from build123d import *

# Parameters (mm, degrees)
SKETCH_R           = 7
PAD_DEPTH          = 61
SKETCH001_R        = 5.425
POCKET_DEPTH       = 61.001
POCKET001_DEPTH    = 5
SKETCH004_W        = 4
SKETCH004_H        = 10
POCKET002_DEPTH    = 5
POLARPATTERN_COUNT = 4


with BuildPart() as part:
    # Sketch → Pad (new body)
    with BuildSketch(Plane.XY):
        Circle(SKETCH_R)
    extrude(amount=PAD_DEPTH)

    # Sketch001 (on Face3 of Pad) → Pocket (cut, through all)
    with BuildSketch(Plane.XY.offset(61)):
        Circle(SKETCH001_R)
    extrude(amount=-POCKET_DEPTH, mode=Mode.SUBTRACT)

    # Sketch002 (on DatumPlane) → Groove (revolve, cut)
    with BuildSketch(Plane(origin=(0, 0, 30.5), x_dir=(0, 0, -1), z_dir=(1, 0, 0))):
        Polygon((-8.25, 9.031089), (-11.75, 9.031089), (-10, 6), align=None)
    revolve(axis=Axis((0, 0, 0), (0, 0, 1)), mode=Mode.SUBTRACT)

    # Sketch003 (on DatumPlane) → Pocket001 (cut)
    with BuildSketch(Plane.YZ.offset(7)):
        Polygon((0, 4.732051), (-1.5, 2.133975), (1.5, 2.133975), align=None)
    extrude(amount=-POCKET001_DEPTH, mode=Mode.SUBTRACT)

    # Sketch004 (on DatumPlane) → Pocket002 (cut)
    with BuildSketch(Plane.YZ.offset(7)):
        with Locations((0, 40.5)):
            Rectangle(SKETCH004_W, SKETCH004_H)
    pocket002 = extrude(amount=-POCKET002_DEPTH, mode=Mode.SUBTRACT)

    # PolarPattern: Pocket002 ×4 about axis
    polarpattern_axis = Axis((0, 0, 0), (0, 0, 1))
    for i in range(1, POLARPATTERN_COUNT):
        add(pocket002.rotate(polarpattern_axis, i * 360 / POLARPATTERN_COUNT), mode=Mode.SUBTRACT)


solid = part.part
Model file for the job. Use its own axes, mm. A direction names the side the tool comes from. Give positions to 0.01 mm unless a question says otherwise; leave off trailing zeros. Write each loop counter-clockwise with the first axis right and the second up, starting at its lowest first coordinate (ties: lowest second). Pieces come first, ordered by that corner, then holes. Notation, with made-up numbers: (27, 62) - (75, 62) arc R13 ccw to (75, 66) - close; hole circle Ø3 at (22.5, 40). An arc over 180 degrees is marked (long way). Answer as CSV lines item,"result".
1. 3-axis set-ups, long thin cutter, end or side, ignore diameter. For faces 4 (the face through (0, 6, 45.5)), 5 (the face through (6, -2, 40)), 6 (the face through (2.503, -4.813, 30.927)): which of +Z, -Z, +X, -X, +Y, -Y reach the whole face in a straight line?
Responses:
face 4,"+Y, -Y"
face 5,"+X, -X"
face 6,"+Z, -Z"
2. Band-saw the part on A-A (x = 0). Write the cut outline in (y, z) (3 decimals), and give its area (3 significant figures).
Responses:
outline,"(-7, 0) - (-5.425, 0) - (-5.425, 35.5) - (-7, 35.5) - close; (-7, 45.5) - (-5.425, 45.5) - (-5.425, 61) - (-7, 61) - close; (5.425, 0) - (7, 0) - (7, 35.5) - (5.425, 35.5) - close; (5.425, 45.5) - (7, 45.5) - (7, 61) - (5.425, 61) - close"
area,"161 mm2"
3. Two-plate mould, pull along Z, no slides. Class faces 1 (the face through (4, -4, 0)), 2 (the face through (6.466, -2.681, 50.899)), 3 (the face through (4.465, 4.403, 40.656)): +Z half, -Z half, draft (parallel to the pull), parting line (faces both ways), or undercut.
Responses:
face 1,"-Z half"
face 2,"draft"
face 3,"undercut"
4. Pin check, flat tips, straight feed: pin 1 (4 mm diameter, centred on y = -4, z = 24.5, fed in from +X); pin 2 (4 mm diameter, centred on x = -5.5, z = 39, fed in from +Y); pin 3 (6 mm diameter, centred on y = -3, z = 18.5, fed in from -X); pin 4 (5 mm diameter, centred on y = -3.5, z = 53.5, fed in from -X). Stop position of each tip, or through.
Responses:
pin 1,"stops at x = 6.71"
pin 2,"stops at y = 6.06"
pin 3,"stops at x = -7"
pin 4,"stops at x = -6.93"
5. Band-saw the part on B-B (z = 55). Write the cut outline in (x, y) (3 decimals).
Responses:
outline,"circle Ø14 at (0, 0); hole circle Ø10.85 at (0, 0)"
6. Drill centre lines: L1, parallel to Y at x = 0, z = 32.5 (3 decimals); L2, parallel to Z at x = 3.25, y = -5.25; L3, parallel to Y at x = 2.25, z = 20. Where is each one in solid material? Low to high. Write a range as [from, to].
Responses:
L1,"y = [-7, -5.425], [5.425, 7]"
L2,"z = [0, 40.4], [40.6, 61]"
L3,"y = [-6.63, -4.94], [4.94, 6.63]"
